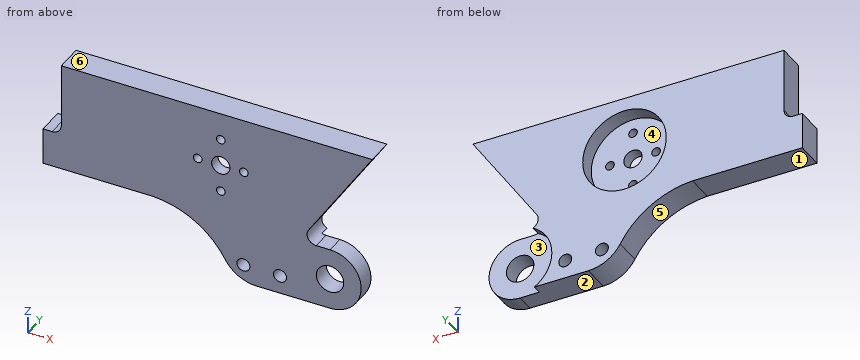
```python
from build123d import *

# Parameters (mm, degrees)
SKETCH1_R           = 4.7625
SKETCH1_R_2         = 2.2479
SKETCH1_R_3         = 1.5
SKETCH1_R_4         = 3.175
BOSS_EXTRUDE1_DEPTH = 9.525
FILLET1_R           = 3.175
FILLET2_R           = 3.175
SKETCH2_R           = 14.5
CUT_EXTRUDE1_DEPTH  = 5.525
SKETCH3_R           = 12.7
CUT_EXTRUDE2_DEPTH  = 3.175


with BuildPart() as part:
    # Sketch1 → Boss-Extrude1 (new body)
    with BuildSketch(Plane(origin=(0, 0, 0), x_dir=(1, 0, 0), z_dir=(0, 1, 0))):
        with BuildLine():
            Line((0, 0), (38.1, 0))
            ThreePointArc((38.1, 0), (52.620300687, 4.403064286), (63.218539249, 15.261399634))
            ThreePointArc((63.218539249, 15.261399634), (67.86863694, 19.924564568), (74.228922018, 21.631986448))
            Line((74.228922018, 21.631986448), (99.628922018, 21.631986448))
            ThreePointArc((99.628922018, 21.631986448), (110.444915242, 10.815993224), (99.628922018, 0))
            Line((99.628922018, 0), (88.9, 0))
            Line((88.9, 0), (114.3, -38.1))
            Line((114.3, -38.1), (6.35, -38.1))
            Line((6.35, -38.1), (6.35, -12.7))
            Line((6.35, -12.7), (0, -12.7))
            Line((0, -12.7), (0, 0))
        make_face()
        with Locations((99.628922018, 10.815993224)):
            Circle(SKETCH1_R, mode=Mode.SUBTRACT)
        with Locations((69.568539249, 15.261399634)):
            Circle(SKETCH1_R_2, mode=Mode.SUBTRACT)
        with Locations((82.268539249, 15.261399634)):
            Circle(SKETCH1_R_2, mode=Mode.SUBTRACT)
        with Locations((69.720479044, -19.05)):
            Circle(SKETCH1_R_3, mode=Mode.SUBTRACT)
        with Locations((61.720479044, -28.55)):
            Circle(SKETCH1_R_3, mode=Mode.SUBTRACT)
        with Locations((53.720479044, -19.05)):
            Circle(SKETCH1_R_3, mode=Mode.SUBTRACT)
        with Locations((61.720479044, -9.55)):
            Circle(SKETCH1_R_3, mode=Mode.SUBTRACT)
        with Locations((61.720479044, -19.05)):
            Circle(SKETCH1_R_4, mode=Mode.SUBTRACT)
    extrude(amount=BOSS_EXTRUDE1_DEPTH)

    # Fillet1
    fillet1_edges = [part.edges().sort_by_distance(p)[0] for p in [
        (88.9, 4.7625, 0),
    ]]
    fillet(fillet1_edges, radius=FILLET1_R)

    # Fillet2
    fillet2_edges = [part.edges().sort_by_distance(p)[0] for p in [
        (6.35, 4.7625, 12.7),
    ]]
    fillet(fillet2_edges, radius=FILLET2_R)

    # Sketch2 → Cut-Extrude1 (cut)
    with BuildSketch(Plane(origin=(0, 9.525, 0), x_dir=(1, 0, 0), z_dir=(0, 1, 0))):
        with Locations((61.720479044, -19.05)):
            Circle(SKETCH2_R)
    extrude(amount=-CUT_EXTRUDE1_DEPTH, mode=Mode.SUBTRACT)

    # Sketch3 → Cut-Extrude2 (cut)
    with BuildSketch(Plane(origin=(0, 9.525, 0), x_dir=(1, 0, 0), z_dir=(0, 1, 0))):
        with Locations((99.628922018, 10.815993224)):
            Circle(SKETCH3_R)
    extrude(amount=-CUT_EXTRUDE2_DEPTH, mode=Mode.SUBTRACT)


solid = part.part
```
Part model, mm, in its own coordinate system. Face numbers are marked on the shaded views. A direction names the side the tool comes from. Give positions to 0.01 mm unless a question says otherwise; leave off trailing zeros. Write each loop counter-clockwise with the first axis right and the second up, starting at its lowest first coordinate (ties: lowest second). Pieces come first, ordered by that corner, then holes. Notation, with made-up numbers: (59.25, 47) -> (114.25, 47) arc R16 cw to (114.25, 60) -> close; hole circle Ø8 at (25.5, -40). An arc over 180 degrees is marked (long way). Put each result on its own line as item: value. Start each with the question number.
Item 1: Pin check, flat tips, straight feed: pin 1 Ø4 at (x, y) = (64.5, 1.5) entering from -Z; pin 2 Ø5 at (x, z) = (61.72, 19.05) entering from +Y; pin 3 Ø5 at (x, z) = (102.5, -13) entering from +Y; pin 4 Ø2 at (x, y) = (55.5, 7.5) entering from -Z. Stop position of each tip, or through.
Item 2: Cut at D-D (y = 2.75). State how many separate pieces and enclosed holes the cut face has, then the cut area to 3 significant figures.
Item 3: Pull direction X, two halves, no side cores. Call the marked faces 4, 5 and 6: pulls with the +X half, pulls with the -X half, needs draft (parallel to the pull), parting line crosses it, or undercut.
Item 4: Which spindle directions (+Z, -Z, +X, -X, +Y, -Y) get a long thin tool onto all of the face, cutting with end or side? Do the marked faces 1, 2 and 3. Say none if no direction does.
Item 5: Cut at A-A (z = 19.05). List the corners of the cut face in (x, y) (3 decimals), then the cut area to 3 significant figures.
Item 6: Cut at B-B (z = 28.55). List the corners of the cut face in (x, y) (3 decimals), then the cut area to 3 significant figures.
Item 7: Wall check: L1, parallel to Z at x = 69, y = 8.5; L2, parallel to X at y = 1.4, z = 19.05; L3, parallel to Z at x = 33, y = 8. Give the ranges that are in metal, low to high. Write a range as [from, to].
Item 8: Cut at C-C (x = 96). List the corners of the cut face in (y, z) (3 decimals).
Answer list:
1. pin 1: stops at z = -19.01
1. pin 2: passes through
1. pin 3: stops at y = 6.35
1. pin 4: stops at z = -7.2
2. separate pieces: 1
2. enclosed holes: 8
2. area: 4,620 mm2
3. face 4: undercut
3. face 5: pulls with the -X half
3. face 6: needs draft
4. face 1: -Z, -X, +Y, -Y
4. face 2: -Z, +X, -X, +Y, -Y
4. face 3: +X, +Y
5. outline: (6.35, 0) -> (52.22, 0) -> (52.22, 4) -> (47.22, 4) -> (47.22, 9.525) -> (6.35, 9.525) -> close; (55.22, 0) -> (58.545, 0) -> (58.545, 4) -> (55.22, 4) -> close; (64.895, 0) -> (68.22, 0) -> (68.22, 4) -> (64.895, 4) -> close; (71.22, 0) -> (101.6, 0) -> (101.6, 9.525) -> (76.22, 9.525) -> (76.22, 4) -> (71.22, 4) -> close
5. area: 698 mm2
6. outline: (6.35, 0) -> (60.22, 0) -> (60.22, 4) -> (50.766, 4) -> (50.766, 9.525) -> (6.35, 9.525) -> close; (63.22, 0) -> (107.933, 0) -> (107.933, 9.525) -> (72.675, 9.525) -> (72.675, 4) -> (63.22, 4) -> close
6. area: 835 mm2
7. L1: z = [-20.51, -17.44], [-13.09, 6.51], [31.59, 38.1]
7. L2: x = [6.35, 52.22], [55.22, 58.55], [64.9, 68.22], [71.22, 101.6]
7. L3: z = [0, 38.1]
8. outline: (0, -21.632) -> (6.35, -21.632) -> (6.35, -13.9) -> (0, -13.9) -> close; (0, -7.732) -> (6.35, -7.732) -> (6.35, 0) -> (0, 0) -> close; (0, 10.65) -> (9.525, 10.65) -> (9.525, 38.1) -> (0, 38.1) -> close
